Job drawing, mm, ordinate dimensions from the low corner. One solid piece. A direction names the side the tool comes from. Round coordinates to 2 decimals unless told otherwise and drop trailing zeros. Write each loop counter-clockwise with the first axis right and the second up, starting at its lowest first coordinate (ties: lowest second). Pieces come first, ordered by that corner, then holes.
1) Saw through at C-C on y = 3. Write the cut outline in (x, z).
2) Pull direction X, two halves, no side cores. Call the marked faces 1, 2 and 3: +X half, -X half, draft (parallel to the pull), parting line (faces both ways), or undercut.
3) Drill centre lines: L1, parallel to X at y = 9, z = 5.75; L2, parallel to X at y = 16, z = 7; L3, parallel to X at y = 30.5, z = 6. Where is each one in solid material? Low to high.
4) Saw through at D-D on y = 36.5. Write the cut outline in (x, z), and give its area (3 significant figures).
5) Which spindle directions (+Z, -Z, +X, -X, +Y, -Y) get a long thin tool onto all of the face, cutting with end or side? Do the marked faces 4, 5 and 6. Say none if no direction does.
6) Flat gauge pins, fed straight in: pin 1 (3 mm diameter, centred on x = 44.5, z = 4, fed in from -Y); pin 2 (3 mm diameter, centred on x = 55, z = 1.5, fed in from -Y). Where does each tip first touch, or does it go through?
7) Saw through at A-A on x = 25.5. Write the cut outline in (y, z), and give its area (3 significant figures).
8) Saw through at B-B on z = 4.5. Write the cut outline in (x, y), and give its area (3 significant figures).
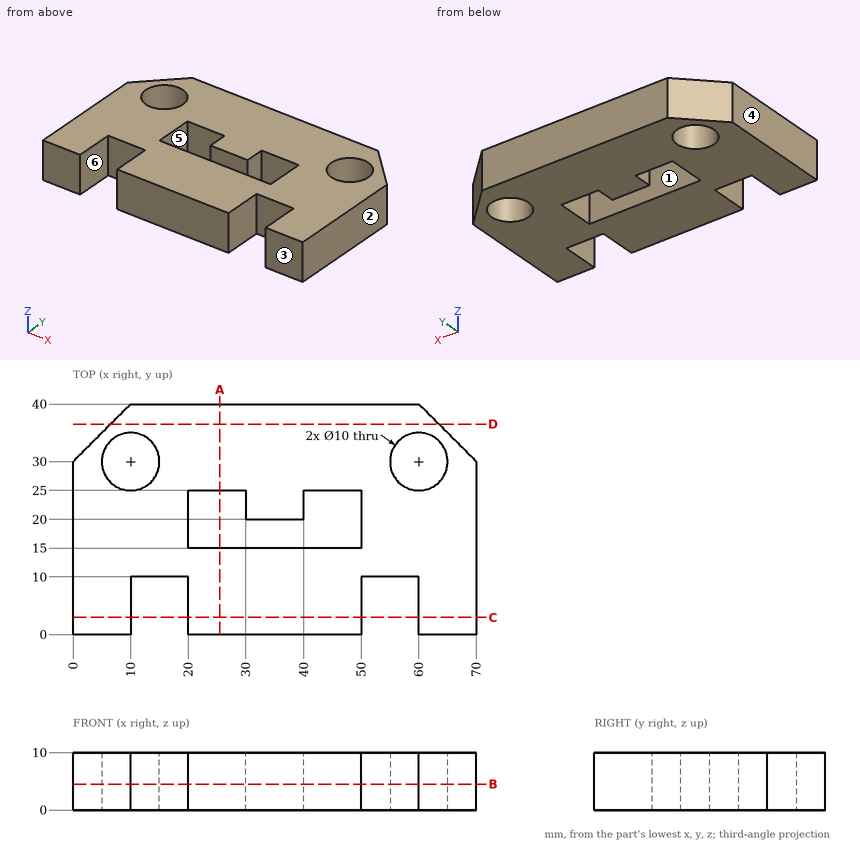
Completed:
1. outline: (0, 0) - (10, 0) - (10, 10) - (0, 10) - close; (20, 0) - (50, 0) - (50, 10) - (20, 10) - close; (60, 0) - (70, 0) - (70, 10) - (60, 10) - close
2. face 1: undercut
2. face 2: +X half
2. face 3: draft
3. L1: x = 0 to 10, 20 to 50, 60 to 70
3. L2: x = 0 to 20, 50 to 70
3. L3: x = 0.5 to 5.03, 14.97 to 55.03, 64.97 to 69.5
4. outline: (6.5, 0) - (63.5, 0) - (63.5, 10) - (6.5, 10) - close
4. area: 570 mm2
5. face 4: +Z, -Z, -X, +Y, -Y
5. face 5: +Z, -Z
5. face 6: +Z, -Z, -Y
6. pin 1: stops at y = 0
6. pin 2: stops at y = 10
7. outline: (0, 0) - (15, 0) - (15, 10) - (0, 10) - close; (25, 0) - (40, 0) - (40, 10) - (25, 10) - close
7. area: 300 mm2
8. outline: (0, 0) - (10, 0) - (10, 10) - (20, 10) - (20, 0) - (50, 0) - (50, 10) - (60, 10) - (60, 0) - (70, 0) - (70, 30) - (60, 40) - (10, 40) - (0, 30) - close; hole circle Ø10 at (10, 30); hole (20, 15) - (50, 15) - (50, 25) - (40, 25) - (40, 20) - (30, 20) - (30, 25) - (20, 25) - close; hole circle Ø10 at (60, 30)
8. area: 2,090 mm2
